The drawing under review shows one solid part. Ordinate dimensions are in mm from its lowest x, y, z. A direction names the side the tool comes from. Coordinates: 2 decimals unless noted, no trailing zeros. Order: outer loops, then holes, each group sorted by start corner. A loop starts at its lowest first (then second) coordinate and runs counter-clockwise, first axis right, second up. Notation, with made-up numbers: (41, -17.75) -> (54, -17.75) arc R29 cw to (54, 18.25) -> close; hole circle Ø4 at (73, -35). An arc over 180 degrees is marked (long way). Put each result on its own line as item: value.
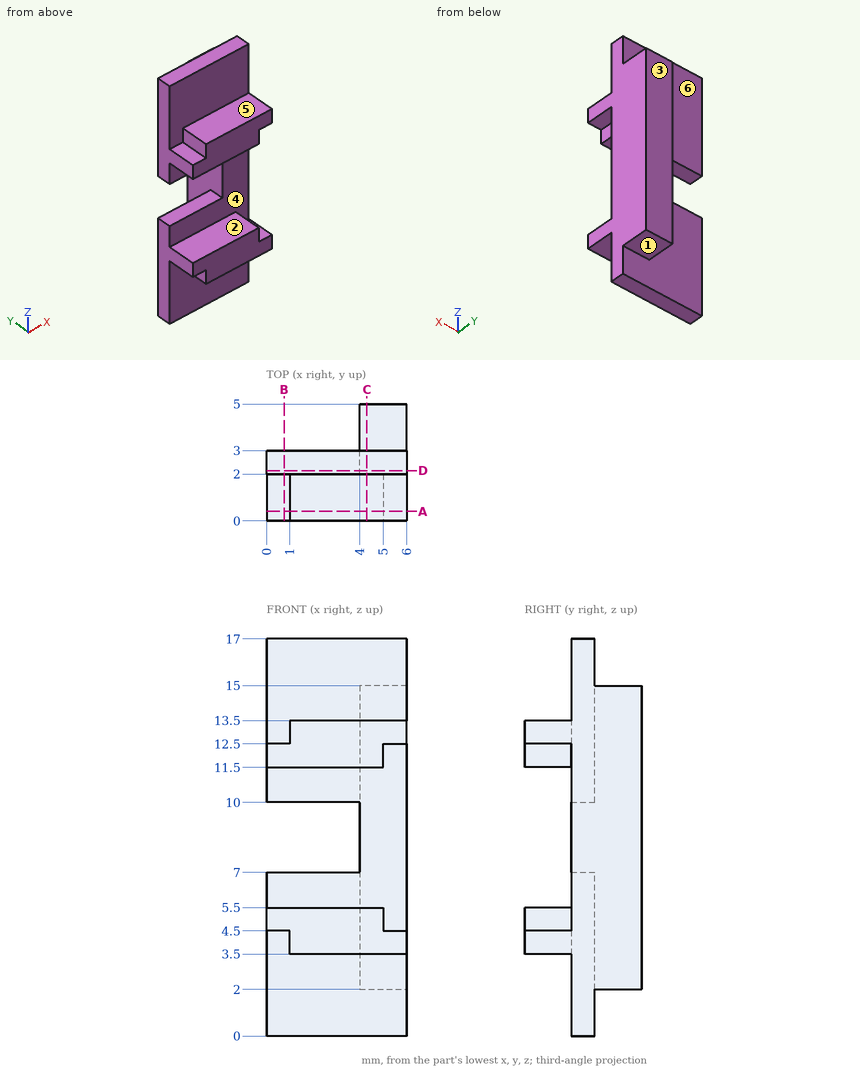
Item 1: Consider section C-C on x = 4.3. Write out the cut boundary in (y, z).
Answers below:
outline: (0, 3.5) -> (2, 3.5) -> (2, 0) -> (3, 0) -> (3, 2) -> (5, 2) -> (5, 15) -> (3, 15) -> (3, 17) -> (2, 17) -> (2, 13.5) -> (0, 13.5) -> (0, 11.5) -> (2, 11.5) -> (2, 5.5) -> (0, 5.5) -> close
Item 2: For pin 1 Ø0.5 at (x, y) = (0.5, 1) entering from +Z; pin 2 Ø0.5 at (y, z) = (1, 5) entering from +X; pin 3 Ø1 at (x, y) = (5, 4) entering from -Z, all flat-tipped, find the tip position at first contact; note any pin that passes through.
Answers below:
pin 1: z = 12.5
pin 2: x = 5
pin 3: z = 2
Item 3: Mouldability with a two-part tool opening along Z and no side actions: class the marked faces 4, 5 and 6 as +Z half, -Z half, draft (parallel to the pull), parting line (faces both ways), or undercut.
Answers below:
face 4: undercut
face 5: +Z half
face 6: draft
Item 4: Consider section B-B on x = 0.75. Write out the cut boundary in (y, z).
Answers below:
outline: (0, 4.5) -> (2, 4.5) -> (2, 0) -> (3, 0) -> (3, 7) -> (2, 7) -> (2, 5.5) -> (0, 5.5) -> close; (0, 11.5) -> (2, 11.5) -> (2, 10) -> (3, 10) -> (3, 17) -> (2, 17) -> (2, 12.5) -> (0, 12.5) -> close
Item 5: Consider section D-D on y = 2.15. Write out the cut boundary in (x, z).
Answers below:
outline: (0, 0) -> (6, 0) -> (6, 17) -> (0, 17) -> (0, 10) -> (4, 10) -> (4, 7) -> (0, 7) -> close
Item 6: For the marked faces 1, 2 and 3, list the 3-axis set-ups (+Z, -Z, +X, -X, +Y, -Y) from which the entire face can be reached by the end or side of a thin tool; tool diameter is ignored.
Answers below:
face 1: -Z, +X, -X, +Y
face 2: +X, -X, -Y
face 3: +Z, -Z, +X, -X, +Y
Item 7: For line 1 (Z direction, x = 0.55, y = 2.95); line 2 (Z direction, x = 2.4, y = 1.15); line 3 (Y direction, x = 2.35, z = 5), list the stretches that pass through material, from the lowest coordinate up. Write a range as from..to.
Answers below:
line 1: 0..7, 10..17
line 2: 3.5..5.5, 11.5..13.5
line 3: 0..3
Item 8: Consider section A-A on y = 0.4. Write out the cut boundary in (x, z), and give its area (3 significant figures).
Answers below:
outline: (0, 4.5) -> (1, 4.5) -> (1, 3.5) -> (6, 3.5) -> (6, 4.5) -> (5, 4.5) -> (5, 5.5) -> (0, 5.5) -> close; (0, 11.5) -> (5, 11.5) -> (5, 12.5) -> (6, 12.5) -> (6, 13.5) -> (1, 13.5) -> (1, 12.5) -> (0, 12.5) -> close
area: 20.0 mm^2
